```python
from build123d import *

# Parameters (mm, degrees)
SKETCH1_W            = 35
SKETCH1_H            = 35
SKETCH1_R            = 6.25
BOSS_EXTRUDE1_DEPTH  = 6
M3_CLEARANCE_HOLE1_D = 3.1


with BuildPart() as part:
    # Sketch1 → Boss-Extrude1 (new body)
    with BuildSketch(Plane(origin=(0, 0, 0), x_dir=(1, 0, 0), z_dir=(0, 1, 0))):
        Rectangle(SKETCH1_W, SKETCH1_H)
        with Locations(Location((0, 0, 0), (0, 0, 270))):
            Circle(SKETCH1_R, mode=Mode.SUBTRACT)
    extrude(amount=BOSS_EXTRUDE1_DEPTH)

    # M3 Clearance Hole1 (through all)
    with Locations(Plane(origin=(0, 6, 0), x_dir=(1, 0, 0), z_dir=(0, 1, 0))):
        with Locations((-13.5, 13.5), (13.5, 13.5), (13.5, -13.5), (-13.5, -13.5), (0, 0)):
            Hole(M3_CLEARANCE_HOLE1_D / 2)


solid = part.part
```
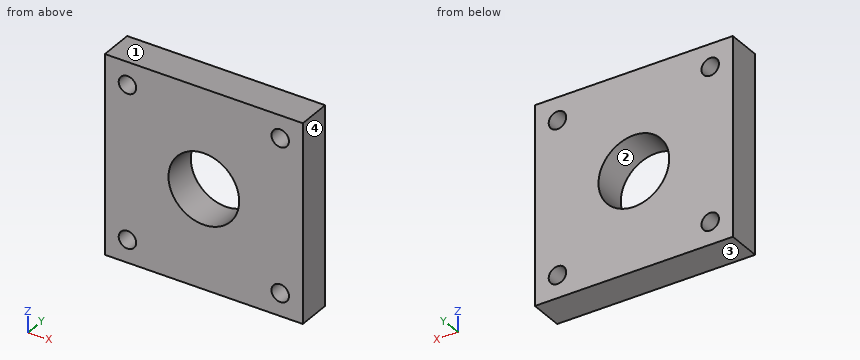
Geometry check sheet. Reference: the model listing, model coordinates, mm. Face numbers are marked on the shaded views. Coordinates: 2 decimals unless noted, no trailing zeros. Write each loop counter-clockwise with the first axis right and the second up, starting at its lowest first coordinate (ties: lowest second). Pieces come first, ordered by that corner, then holes. Notation, with made-up numbers: M 44,72.25 L 67,72.25 A13 ccw 67,78.25 Z; hole C -8,21.5 d1. An arc over 180 degrees is marked long. Answer as a JSON object with one key per item and string values.
1. Section check C-C, the plane y = 3.6. Enter the section's corners in (x, z).
Answers below:
{"outline": "M -17.5,-17.5 L 17.5,-17.5 L 17.5,17.5 L -17.5,17.5 Z; hole C -13.5,-13.5 d3.1; hole C -13.5,13.5 d3.1; hole C 0,0 d12.5; hole C 13.5,-13.5 d3.1; hole C 13.5,13.5 d3.1"}
2. Section check D-D, the plane x = -13.5. Enter the section's corners in (y, z).
Answers below:
{"outline": "M 0,-17.5 L 6,-17.5 L 6,-15.05 L 0,-15.05 Z; M 0,-11.95 L 6,-11.95 L 6,11.95 L 0,11.95 Z; M 0,15.05 L 6,15.05 L 6,17.5 L 0,17.5 Z"}
3. Section check A-A, the plane x = -5. Enter the section's corners in (y, z).
Answers below:
{"outline": "M 0,-17.5 L 6,-17.5 L 6,-3.75 L 0,-3.75 Z; M 0,3.75 L 6,3.75 L 6,17.5 L 0,17.5 Z"}
4. Section check B-B, the plane z = 0. Enter the section's corners in (x, y), plus the area to 3 significant figures.
Answers below:
{"outline": "M -17.5,0 L -6.25,0 L -6.25,6 L -17.5,6 Z; M 6.25,0 L 17.5,0 L 17.5,6 L 6.25,6 Z", "area": "135 mm²"}
5. Scan lines: L1, parallel to Z at x = 13.5, y = 1.5; L2, parallel to X at y = 4.85, z = 14.5. Record each from-to range of solid material in increasing order.
Answers below:
{"L1": "z = -17.5 to -15.05, -11.95 to 11.95, 15.05 to 17.5", "L2": "x = -17.5 to -14.68, -12.32 to 12.32, 14.68 to 17.5"}
6. Draft check along Z on the marked faces 1, 2, 3 and 4. Enter one of: released by +Z, released by -Z, zero draft, split by the parting line, or undercut.
Answers below:
{"face 1": "released by +Z", "face 2": "undercut", "face 3": "released by -Z", "face 4": "zero draft"}
